Job drawing, mm, ordinate dimensions from the low corner. One solid piece. A direction names the side the tool comes from. Round coordinates to 2 decimals unless told otherwise and drop trailing zeros. Loops run counter-clockwise (first coordinate to the right, second up) from the corner with the lowest first, then second, coordinate; pieces in that order, holes last.
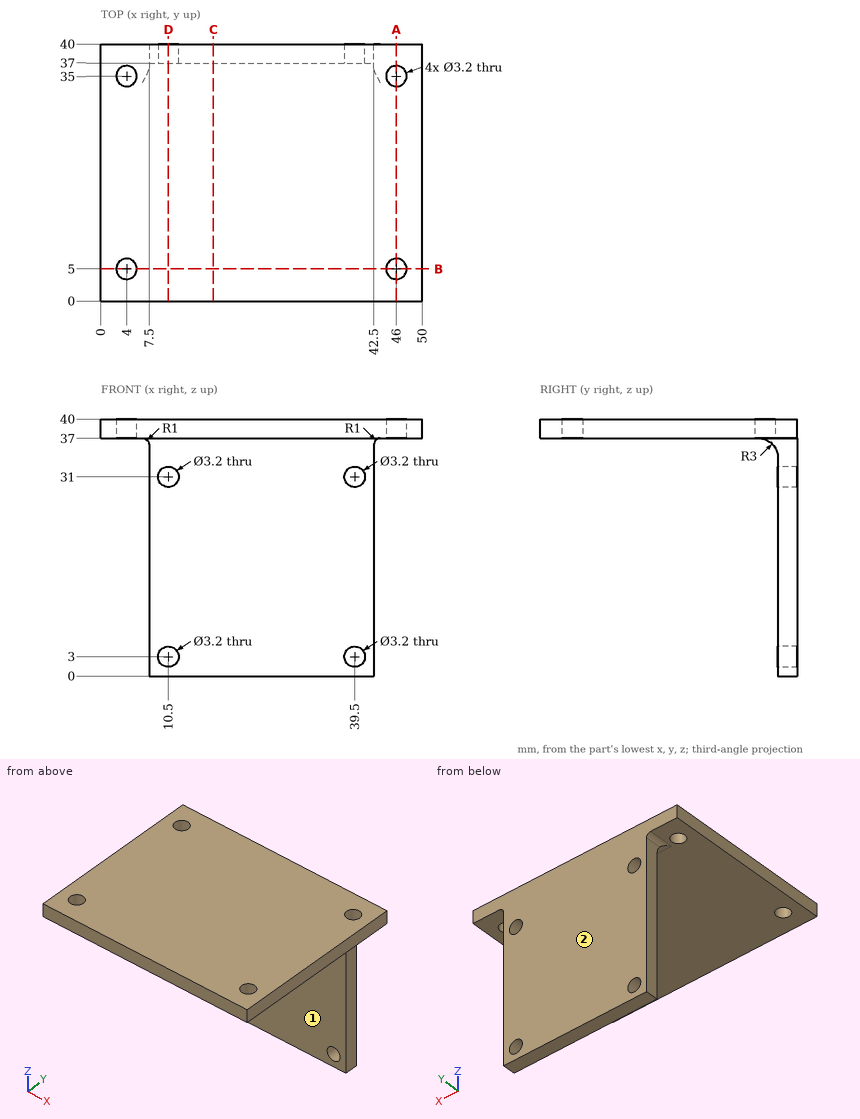
1) Slice it at C-C, the plane x = 17.5. Give the cut face in (y, z), then the cut area to 3 significant figures.
Values:
outline: (0, 37) - (34, 37) arc R3 cw to (37, 34) - (37, 0) - (40, 0) - (40, 40) - (0, 40) - close
area: 233 mm2
2) Wall check: line 1 along Y through (x, z) = (46, 39); line 2 along Z through (x, y) = (10.5, 39.2); line 3 along X through (y, z) = (38.25, 31). Give the ranges that are in metal, low to high.
Values:
line 1: y = 0 to 3.4, 6.6 to 33.4, 36.6 to 40
line 2: z = 0 to 1.4, 4.6 to 29.4, 32.6 to 40
line 3: x = 7.5 to 8.9, 12.1 to 37.9, 41.1 to 42.5
3) Tool access for the marked faces 1 and 2: list every direction of +Z, -Z, +X, -X, +Y, -Y with a clear straight run to the whole face (end or side of a thin tool).
Values:
face 1: -Z, +X, -X, -Y
face 2: +Z, -Z, +X, -X, +Y
4) Drop flat-ended pins along their axis: pin 1 Ø5 at (x, z) = (39.5, 31) entering from -Y; pin 2 Ø1.9 at (x, z) = (39.5, 3) entering from -Y; pin 3 Ø1.1 at (y, z) = (37.5, 26) entering from +X; pin 4 Ø12 at (x, y) = (28, 25.5) entering from -Z. Give the stop position or say it passes through.
Values:
pin 1: stops at y = 37
pin 2: passes through
pin 3: stops at x = 42.5
pin 4: stops at z = 37
5) Slice it at B-B, the plane y = 5. Give the cut face in (x, z), then the cut area to 3 significant figures.
Values:
outline: (0, 37) - (2.4, 37) - (2.4, 40) - (0, 40) - close; (5.6, 37) - (44.4, 37) - (44.4, 40) - (5.6, 40) - close; (47.6, 37) - (50, 37) - (50, 40) - (47.6, 40) - close
area: 131 mm2
6) Slice it at D-D, the plane x = 10.5. Give the cut face in (y, z), then the cut area to 3 significant figures.
Values:
outline: (0, 37) - (34, 37) arc R3 cw to (37, 34) - (37, 32.6) - (40, 32.6) - (40, 40) - (0, 40) - close; (37, 0) - (40, 0) - (40, 1.4) - (37, 1.4) - close; (37, 4.6) - (40, 4.6) - (40, 29.4) - (37, 29.4) - close
area: 214 mm2
7) Slice it at A-A, the plane x = 46. Give the cut face in (y, z), then the cut area to 3 significant figures.
Values:
outline: (0, 37) - (3.4, 37) - (3.4, 40) - (0, 40) - close; (6.6, 37) - (33.4, 37) - (33.4, 40) - (6.6, 40) - close; (36.6, 37) - (40, 37) - (40, 40) - (36.6, 40) - close
area: 101 mm2
